Autodesk Fusion 360 part; units mm, degrees
sketch "Sketch1" plane through (0, 0, 0) normal (0, 0, 1) x (1, 0, 0)
  line L0 (0, 0) -> (53.2, 0)
  line L1 (53.2, 0) -> (53.2, 40.2)
  line L2 (53.2, 40.2) -> (0, 40.2)
  line L3 (0, 40.2) -> (0, 0)
  circle A0 centre (4.6, 4.6) radius 1.75
  circle A1 centre (4.6, 35.6) radius 1.75
  circle A2 centre (48.6, 35.6) radius 1.75
  circle A3 centre (48.6, 4.6) radius 1.75
  dimension "d1" = 53.2
  dimension "d2" = 40.2
  dimension "d3" = 4.6
  dimension "d4" = 4.6
  dimension "d5" = 4.6
  dimension "d6" = 4.6
  dimension "d7" = 4.6
  dimension "d8" = 4.6
  dimension "d9" = 4.6
  dimension "d10" = 4.6
  dimension "d11" = 3.5
  dimension "d12" = 3.5
  dimension "d13" = 3.5
  dimension "d14" = 3.5
extrude "Extrude1" add sketch "Sketch1" along normal blind 4
fillet "Fillet1" radius 4.6 4 edges at (0, 40.2, 2) (0, 0, 2) (53.2, 0, 2) (53.2, 40.2, 2)
sketch "Sketch2" plane through (0, 0, 0) normal (0, 0, -1) x (-1, 0, 0)
  arc A0 (-48.6, 40.2) -> (-53.2, 35.6) centre (-48.6, 35.6) ccw
  line L0 (-53.2, 35.6) -> (-53.2, 4.6)
  arc A1 (-53.2, 4.6) -> (-48.6, 0) centre (-48.6, 4.6) ccw
  line L1 (-48.6, 0) -> (-4.6, 0)
  arc A2 (-4.6, 0) -> (0, 4.6) centre (-4.6, 4.6) ccw
  line L2 (0, 4.6) -> (0, 35.6)
  arc A3 (0, 35.6) -> (-4.6, 40.2) centre (-4.6, 35.6) ccw
  line L3 (-4.6, 40.2) -> (-48.6, 40.2)
  circle A4 centre (-48.6, 4.6) radius 1.75
  circle A5 centre (-48.6, 35.6) radius 1.75
  circle A6 centre (-4.6, 4.6) radius 1.75
  circle A7 centre (-4.6, 35.6) radius 1.75
  line L4 (-51.6, 35.6) -> (-51.6, 4.6)
  arc A8 (-51.6, 4.6) -> (-48.6, 1.6) centre (-48.6, 4.6) ccw
  line L5 (-48.6, 1.6) -> (-4.6, 1.6)
  arc A9 (-4.6, 1.6) -> (-1.6, 4.6) centre (-4.6, 4.6) ccw
  line L6 (-1.6, 4.6) -> (-1.6, 35.6)
  arc A10 (-1.6, 35.6) -> (-4.6, 38.6) centre (-4.6, 35.6) ccw
  line L7 (-4.6, 38.6) -> (-48.6, 38.6)
  arc A11 (-48.6, 38.6) -> (-51.6, 35.6) centre (-48.6, 35.6) ccw
  dimension "d18" = 1.6
extrude "Extrude2" cut sketch "Sketch2" against normal blind 2 contours L4 A8 L5 A9 L6 A10 L7 A11
sketch "Sketch3" plane through (0, 0, 0) normal (0, 0, -1) x (-1, 0, 0)
  line L0 (-51.6, 4.6) -> (-51.6, 35.6)
  arc A0 (-48.6, 38.6) -> (-51.6, 35.6) centre (-48.6, 35.6) ccw
  line L1 (-48.6, 38.6) -> (-4.6, 38.6)
  arc A1 (-1.6, 35.6) -> (-4.6, 38.6) centre (-4.6, 35.6) ccw
  line L2 (-1.6, 35.6) -> (-1.6, 4.6)
  arc A2 (-4.6, 1.6) -> (-1.6, 4.6) centre (-4.6, 4.6) ccw
  line L3 (-4.6, 1.6) -> (-48.6, 1.6)
  arc A3 (-51.6, 4.6) -> (-48.6, 1.6) centre (-48.6, 4.6) ccw
  arc A4 (-48.6, 40.2) -> (-53.2, 35.6) centre (-48.6, 35.6) ccw
  line L4 (-53.2, 35.6) -> (-53.2, 4.6)
  arc A5 (-53.2, 4.6) -> (-48.6, 0) centre (-48.6, 4.6) ccw
  line L5 (-48.6, 0) -> (-4.6, 0)
  arc A6 (-4.6, 0) -> (0, 4.6) centre (-4.6, 4.6) ccw
  line L6 (0, 4.6) -> (0, 35.6)
  arc A7 (0, 35.6) -> (-4.6, 40.2) centre (-4.6, 35.6) ccw
  line L7 (-4.6, 40.2) -> (-48.6, 40.2)
  line L8 (0, 24.6) -> (-1.6, 24.6)
  line L9 (0, 7.6) -> (-1.6, 7.6)
  line L10 (-53.2, 28.6) -> (-51.6, 28.6)
  line L11 (-53.2, 6.6) -> (-51.6, 6.6)
  line L12 (-46.35, 40.2) -> (-46.35, 38.6)
  line L13 (-7.35, 40.2) -> (-7.35, 38.6)
  dimension "d21" = 17
  dimension "d22" = 11
  dimension "d25" = 5
  dimension "d26" = 10
  dimension "d27" = 5.75
  dimension "d73" = 39
extrude "Extrude3" cut sketch "Sketch3" against normal blind 2 contours L0 L4 L10 L11 | L2 L6 L8 L9 | L1 L7 L12 L13
sketch "Sketch4" plane through (0, 0, 2) normal (0, 0, -1) x (-1, 0, 0)
  circle A0 centre (-48.6, 4.6) radius 1.75
  circle A1 centre (-4.6, 35.6) radius 1.75
  circle A2 centre (-4.6, 4.6) radius 1.75
  circle A3 centre (-48.6, 35.6) radius 1.75
  line L0 (-53.2, 28.6) -> (-53.2, 6.6)
  line L1 (0, 7.6) -> (0, 24.6)
  line L2 (-7.35, 40.2) -> (-46.35, 40.2)
  arc A4 (-48.6, 38.6) -> (-51.6, 35.6) centre (-48.6, 35.6) ccw
  line L3 (-51.6, 35.6) -> (-51.6, 28.6)
  line L4 (-51.6, 28.6) -> (-53.2, 28.6)
  line L5 (-53.2, 6.6) -> (-51.6, 6.6)
  line L6 (-51.6, 6.6) -> (-51.6, 4.6)
  arc A5 (-51.6, 4.6) -> (-48.6, 1.6) centre (-48.6, 4.6) ccw
  line L7 (-48.6, 1.6) -> (-4.6, 1.6)
  arc A6 (-4.6, 1.6) -> (-1.6, 4.6) centre (-4.6, 4.6) ccw
  line L8 (-1.6, 4.6) -> (-1.6, 7.6)
  line L9 (-1.6, 7.6) -> (0, 7.6)
  line L10 (0, 24.6) -> (-1.6, 24.6)
  line L11 (-1.6, 24.6) -> (-1.6, 35.6)
  arc A7 (-1.6, 35.6) -> (-4.6, 38.6) centre (-4.6, 35.6) ccw
  line L12 (-4.6, 38.6) -> (-7.35, 38.6)
  line L13 (-7.35, 38.6) -> (-7.35, 40.2)
  line L14 (-46.35, 40.2) -> (-46.35, 38.6)
  line L15 (-46.35, 38.6) -> (-48.6, 38.6)
  line L16 (-51.6, 28.6) -> (-45.1, 28.6)
  line L17 (-45.1, 28.6) -> (-45.1, 6.6)
  line L18 (-45.1, 6.6) -> (-51.6, 6.6)
  line L19 (-7.35, 38.6) -> (-7.35, 31.6)
  line L20 (-7.35, 31.6) -> (-46.35, 31.6)
  line L21 (-46.35, 31.6) -> (-46.35, 38.6)
  line L22 (-1.6, 24.6) -> (-6.6, 24.6)
  line L23 (-6.6, 24.6) -> (-6.6, 7.6)
  line L24 (-6.6, 7.6) -> (-1.6, 7.6)
  line L25 (-12.1, 1.6) -> (-12.1, 8.6)
  line L26 (-12.1, 8.6) -> (-23.6, 8.6)
  line L27 (-23.6, 8.6) -> (-23.6, 1.6)
  line L28 (-25.1, 1.6) -> (-25.1, 6.1)
  line L29 (-25.1, 6.1) -> (-43.6, 6.1)
  line L30 (-43.6, 6.1) -> (-43.6, 1.6)
  dimension "d74" = 6.5
  dimension "d75" = 7
  dimension "d76" = 5
  dimension "d77" = 10.5
  dimension "d78" = 11.5
  dimension "d79" = 7
  dimension "d80" = 4.5
  dimension "d81" = 23.5
  dimension "d82" = 18.5
extrude "Extrude4" cut sketch "Sketch4" against normal blind 2 contours L0 L4 L5 L16 L17 L18 | L2 L13 L14 L19 L20 L21 | L7 L28 L29 L30 | L7 L25 L26 L27 | L1 L9 L10 L22 L23 L24
sketch "Sketch5" plane through (0, 0, 2) normal (0, 0, -1) x (-1, 0, 0)
  line L0 (-51.6, 35.6) -> (-51.6, 28.6)
  line L1 (-48.6, 1.6) -> (-43.6, 1.6)
  line L2 (-1.6, 7.6) -> (-6.6, 7.6)
  line L3 (-6.6, 24.6) -> (-1.6, 24.6)
  line L4 (-7.35, 38.6) -> (-7.35, 31.6)
  line L5 (-4.6, 38.6) -> (-7.35, 38.6)
  line L6 (-46.35, 31.6) -> (-46.35, 38.6)
  line L7 (-51.6, 28.6) -> (-45.1, 28.6)
  line L8 (-45.1, 6.6) -> (-51.6, 6.6)
  circle A0 centre (-48.6, 35.6) radius 1.75
  circle A1 centre (-4.6, 4.6) radius 1.75
  circle A2 centre (-4.6, 35.6) radius 1.75
  circle A3 centre (-48.6, 4.6) radius 1.75
  line L9 (-12.6, 8.6) -> (-6.6, 8.6)
  line L10 (-6.6, 8.6) -> (-6.6, 2.6)
  line L11 (-6.6, 2.6) -> (-12.6, 2.6)
  line L12 (-12.6, 2.6) -> (-12.6, 8.6)
  arc A4 (-4.6, 1.6) -> (-1.6, 4.6) centre (-4.6, 4.6) ccw
  line L13 (-1.6, 4.6) -> (-1.6, 7.6)
  line L14 (-1.6, 24.6) -> (-1.6, 35.6)
  arc A5 (-1.6, 35.6) -> (-4.6, 38.6) centre (-4.6, 35.6) ccw
  line L15 (-46.35, 38.6) -> (-48.6, 38.6)
  arc A6 (-48.6, 38.6) -> (-51.6, 35.6) centre (-48.6, 35.6) ccw
  line L16 (-51.6, 6.6) -> (-51.6, 4.6)
  arc A7 (-51.6, 4.6) -> (-48.6, 1.6) centre (-48.6, 4.6) ccw
  line L17 (-45.1, 28.6) -> (-45.1, 6.6)
  line L18 (-43.6, 1.6) -> (-43.6, 6.1)
  line L19 (-43.6, 6.1) -> (-25.1, 6.1)
  line L20 (-25.1, 6.1) -> (-25.1, 1.6)
  line L21 (-25.1, 1.6) -> (-23.6, 1.6)
  line L22 (-23.6, 1.6) -> (-23.6, 8.6)
  line L23 (-23.6, 8.6) -> (-12.1, 8.6)
  line L24 (-12.1, 8.6) -> (-12.1, 1.6)
  line L25 (-12.1, 1.6) -> (-4.6, 1.6)
  line L26 (-6.6, 7.6) -> (-6.6, 24.6)
  line L27 (-7.35, 31.6) -> (-46.35, 31.6)
  dimension "d49" = 6
  dimension "d51" = 6
  dimension "d83" = 1
  dimension "d84" = 5
extrude "Extrude5" cut sketch "Sketch5" against normal blind 1.3 contours L9 L10 L11 L24 L26 | L9 L11 L12 L23 L24
sketch "Sketch8" plane through (0, 0, 2) normal (0, 0, -1) x (-1, 0, 0)
  line L0 (-6.6, 24.6) -> (-1.6, 24.6)
  line L1 (-7.35, 38.6) -> (-7.35, 31.6)
  line L2 (-4.6, 38.6) -> (-7.35, 38.6)
  line L3 (-46.35, 31.6) -> (-46.35, 38.6)
  line L4 (-51.6, 28.6) -> (-45.1, 28.6)
  line L5 (-45.1, 6.6) -> (-51.6, 6.6)
  line L6 (-51.6, 35.6) -> (-51.6, 28.6)
  line L7 (-48.6, 1.6) -> (-43.6, 1.6)
  line L8 (-23.6, 8.6) -> (-6.6, 8.6)
  circle A0 centre (-48.6, 35.6) radius 1.75
  circle A1 centre (-4.6, 35.6) radius 1.75
  circle A2 centre (-48.6, 4.6) radius 1.75
  arc A3 (-1.6, 35.6) -> (-4.6, 38.6) centre (-4.6, 35.6) ccw
  line L9 (-46.35, 38.6) -> (-48.6, 38.6)
  arc A4 (-48.6, 38.6) -> (-51.6, 35.6) centre (-48.6, 35.6) ccw
  line L10 (-51.6, 6.6) -> (-51.6, 4.6)
  arc A5 (-51.6, 4.6) -> (-48.6, 1.6) centre (-48.6, 4.6) ccw
  line L11 (-6.6, 8.6) -> (-6.6, 24.6)
  line L12 (-7.35, 31.6) -> (-46.35, 31.6)
  line L13 (-45.1, 28.6) -> (-45.1, 6.6)
  line L14 (-43.6, 1.6) -> (-43.6, 6.1)
  line L15 (-43.6, 6.1) -> (-25.1, 6.1)
  line L16 (-25.1, 6.1) -> (-25.1, 1.6)
  line L17 (-25.1, 1.6) -> (-23.6, 1.6)
  line L18 (-23.6, 1.6) -> (-23.6, 8.6)
  line L19 (-1.6, 24.6) -> (-1.6, 35.6)
  line L20 (-45.1, 6.6) -> (-43.6, 6.1)
  line L21 (-7.35, 31.6) -> (-1.6, 31.6)
  line L22 (-46.35, 31.6) -> (-46.6643, 31.6)
  line L23 (-46.6643, 31.6) -> (-51.6, 31.6)
  line L24 (-6.6, 7.6) -> (-6.6, 2.6)
  line L25 (-6.6, 2.6) -> (-12.1, 2.6)
  line L26 (-12.1, 2.6) -> (-12.1, 1.6)
  line L27 (-12.1, 1.6) -> (-4.6, 1.6)
  arc A6 (-4.6, 1.6) -> (-1.6, 4.6) centre (-4.6, 4.6) ccw
  line L28 (-1.6, 4.6) -> (-1.6, 7.6)
  line L29 (-1.6, 7.6) -> (-6.6, 7.6)
  circle A7 centre (-4.6, 4.6) radius 1.75
  line L30 (-6.6, 2.6) -> (-6.6, 1.6)
extrude "Extrude8" add sketch "Sketch8" along normal blind 2 contours L1 L2 A3 L19 L21 | L3 L6 L9 A4 L22 L23 | L5 L7 L10 A5 L14 L20 | L24 L27 A6 L28 L29 L30
sketch "Sketch9" plane through (0, 0, 2) normal (0, 0, -1) x (-1, 0, 0)
  line L0 (-45.1, 6.6) -> (-43.6, 6.1)
  line L1 (-43.6, 6.1) -> (-25.1, 6.1)
  line L2 (-25.1, 6.1) -> (-25.1, 1.6)
  line L3 (-25.1, 1.6) -> (-23.6, 1.6)
  line L4 (-23.6, 1.6) -> (-23.6, 8.6)
  line L5 (-23.6, 8.6) -> (-6.6, 8.6)
  line L6 (-6.6, 8.6) -> (-6.6, 24.6)
  line L7 (-6.6, 24.6) -> (-1.6, 24.6)
  line L8 (-1.6, 24.6) -> (-1.6, 31.6)
  line L9 (-1.6, 31.6) -> (-7.35, 31.6)
  line L10 (-7.35, 31.6) -> (-46.35, 31.6)
  line L11 (-46.35, 31.6) -> (-51.6, 31.6)
  line L12 (-51.6, 31.6) -> (-51.6, 28.6)
  line L13 (-51.6, 28.6) -> (-45.1, 28.6)
  line L14 (-45.1, 28.6) -> (-45.1, 6.6)
  line L15 (-7.6, 10.6) -> (-9.6, 10.6)
  line L16 (-9.6, 10.6) -> (-9.6, 13.6)
  line L17 (-9.6, 13.6) -> (-7.6, 13.6)
  line L18 (-7.6, 13.6) -> (-7.6, 10.6)
  dimension "d85" = 2
  dimension "d86" = 1
  dimension "d87" = 3
  dimension "d88" = 2
extrude "Extrude9" cut sketch "Sketch9" against normal blind 1.5 contours L15 L16 L17 L18
equation "d1 = 50 mm + ( ( 2 * 1.6 ) * 1 mm )"
equation "d2 = 37 mm + ( ( 2 * 1.6 ) * 1 mm )"
equation "d3 = 3 mm + 1.6 mm"
equation "d4 = d3"
equation "d5 = d4"
equation "d6 = d3"
equation "d7 = d3"
equation "d8 = d7"
equation "d9 = d4"
equation "d10 = d5"
equation "d17 = 3 mm + 1.6 mm"
Could you check a few things on this model? Use its own coordinates, in mm. A direction names the side the tool comes from. Coordinates: 2 decimals unless noted, no trailing zeros. Write each loop counter-clockwise with the first axis right and the second up, starting at its lowest first coordinate (ties: lowest second). Pieces come first, ordered by that corner, then holes. Notation, with made-up numbers: M 7,31 L 51,31 A32 ccw 51,69 Z; hole C -37,5 d1. An arc over 180 degrees is marked long. Answer as CSV lines item,"result". Start each with the question number.
1) For faces 1 (the flat face through (9, 12, 3.5)), 2 (the flat face through (44.36, 6.353, 1.014)), 3 (the flat face through (6.6, 16, 3)), which set-ups out of +Z, -Z, +X, -X, +Y, -Y let a thin tool reach every point of the face, with its end or its side?
2) We'd pull the mould along X, two halves only. Please class faces 4 (the cylindrical face through (51.817, 1.312, 2.028)), 5 (the flat face through (6, 40.2, 2)), 6 (the flat face through (6.6, 5, 2)): +X half, -X half, draft (parallel to the pull), parting line (faces both ways), or undercut.
3) I want a section at D-D, the plane y = 27. Please give me the cut outline in (x, z).
4) Please list where these lines run through material, in increasing order: line 1 (X direction, y = 4.5, z = 1.35); line 2 (X direction, y = 35.6, z = 1.55); line 3 (Y direction, x = 4.6, z = 3.3). Write a range as from..to.
5) I want a section at B-B, the plane x = 16. Please give me the cut outline in (y, z).
6) For P1, Ø0.8, axis at y = 12, z = 3, coming from the +X side; P2, Ø8, axis at x = 21.5, y = 25.5, coming from the -Z side; P3, Ø2, axis at y = 37.5, z = 1.5, coming from the -X side; P4, Ø5.5, axis at x = 48.6, y = 4.6, coming from the -Z side, each with a flat end and sliding along its axis, tell me the tip position at first contact or that it passes through.
7) I want a section at C-C, the plane x = 24.5. Please give me the cut outline in (y, z), and give its area (3 significant figures).
8) I want a section at A-A, the plane z = 0.65. Give the number of separate pieces and of enclosed holes in the cut face, and give its area (3 significant figures).
Data:
1,face 1,"-Z"
1,face 2,"-Z, +Y"
1,face 3,"+Z, -Z, -X"
2,face 4,"+X half"
2,face 5,"draft"
2,face 6,"undercut"
3,outline,"M 0,0 L 1.6,0 L 1.6,2 L 45.1,2 L 45.1,4 L 0,4 Z"
4,line 1,"x = 0..2.85, 6.35..6.6, 43.6..46.85, 50.35..53.2"
4,line 2,"x = 0..2.85, 6.35..7.35, 46.35..46.85, 50.35..53.2"
4,line 3,"y = 0..2.85, 6.35..7.6, 24.6..33.85, 37.35..40.2"
5,outline,"M 0,0 L 1.6,0 L 1.6,4 L 0,4 Z; M 8.6,2 L 31.6,2 L 31.6,4 L 8.6,4 Z"
6,P1,"stops at x = 45.1"
6,P2,"stops at z = 2"
6,P3,"stops at x = 0.09"
6,P4,"stops at z = 0"
7,outline,"M 0,0 L 1.6,0 L 1.6,2 L 31.6,2 L 31.6,4 L 0,4 Z"
7,area,"66.4 mm^2"
8,separate pieces,"3"
8,enclosed holes,"4"
8,area,"254 mm^2"
